```python
from build123d import *

# Parameters (mm, degrees)
SKETCH1_W           = 71.7
SKETCH1_H           = 101.4
BOSS_EXTRUDE1_DEPTH = 11.1
SKETCH5_W           = 87
SKETCH5_H           = 14.461590439
CUT_EXTRUDE1_DEPTH  = 64.5
FILLET2_R           = 1
SKETCH7_R           = 1.5
CUT_EXTRUDE3_DEPTH  = 4
SKETCH10_W          = 8.724930765
SKETCH10_H          = 5.55
CUT_EXTRUDE5_DEPTH  = 10
SKETCH11_W          = 7.2
SKETCH11_H          = 5.55
BOSS_EXTRUDE2_DEPTH = 10
FILLET3_R           = 0.5


with BuildPart() as part:
    # Sketch1 → Boss-Extrude1 (new body)
    with BuildSketch(Plane(origin=(0, 0, 0), x_dir=(1, 0, 0), z_dir=(0, 1, 0))):
        Rectangle(SKETCH1_W, SKETCH1_H)
    extrude(amount=BOSS_EXTRUDE1_DEPTH)

    # Sketch5 → Cut-Extrude1 (cut)
    with BuildSketch(Plane(origin=(35.85, 0, 0), x_dir=(0, 0, -1), z_dir=(1, 0, 0))):
        with Locations((0, 11.23079522)):
            Rectangle(SKETCH5_W, SKETCH5_H)
    extrude(amount=-CUT_EXTRUDE1_DEPTH, mode=Mode.SUBTRACT)

    # Fillet2
    fillet2_edges = [part.edges().sort_by_distance(p)[0] for p in [
        (0, 11.1, -50.7),
        (-35.85, 11.1, 0),
        (-35.85, 0, 0),
        (0, 11.1, 50.7),
        (-35.85, 5.55, -50.7),
        (-35.85, 5.55, 50.7),
    ]]
    fillet(fillet2_edges, radius=FILLET2_R)

    # Sketch7 → Cut-Extrude3 (cut)
    with BuildSketch(Plane(origin=(0, 11.1, 0), x_dir=(1, 0, 0), z_dir=(0, 1, 0))):
        with Locations(Location((-31.75, -6.65790951, 0), (0, 0, 270))):
            Circle(SKETCH7_R)
        with Locations(Location((-31.75, 6.65790951, 0), (0, 0, 90))):
            Circle(SKETCH7_R)
    extrude(amount=-CUT_EXTRUDE3_DEPTH, mode=Mode.SUBTRACT)

    # Sketch10 → Cut-Extrude5 (cut)
    with BuildSketch(Plane(origin=(35.85, 0, 0), x_dir=(0, 0, -1), z_dir=(1, 0, 0))):
        with Locations((-47.862465383, 8.325)):
            Rectangle(SKETCH10_W, SKETCH10_H)
    extrude(amount=-CUT_EXTRUDE5_DEPTH, mode=Mode.SUBTRACT)

    # Sketch11 → Boss-Extrude2 (add)
    with BuildSketch(Plane(origin=(35.85, 0, 0), x_dir=(0, 0, -1), z_dir=(1, 0, 0))):
        with Locations((47.1, 2.775)):
            Rectangle(SKETCH11_W, SKETCH11_H)
    extrude(amount=BOSS_EXTRUDE2_DEPTH)

    # Fillet3
    fillet3_edges = [part.edges().sort_by_distance(p)[0] for p in [
        (-28.65, 4, 0),
        (3.6, 4, -43.5),
        (3.6, 4, 43.5),
        (-28.65, 7.55, -43.5),
        (-28.65, 7.55, 43.5),
        (25.85, 5.55, 47.1),
        (35.85, 5.55, -47.1),
        (35.85, 2, -43.5),
    ]]
    fillet(fillet3_edges, radius=FILLET3_R)


solid = part.part
```
Geometry check sheet. Reference: the model listing, model coordinates, mm. A direction names the side the tool comes from. Give positions to 0.01 mm unless a question says otherwise; leave off trailing zeros. Write each loop counter-clockwise with the first axis right and the second up, starting at its lowest first coordinate (ties: lowest second). Pieces come first, ordered by that corner, then holes.
1) Release check for a two-part mould opening along Z. For faces 1 (the flat face through (-32, 7.1, 7)), 2 (the flat face through (5, 0, 1)), 3 (the flat face through (8, 8, -43.5)), 4 (the flat face through (5, 5, -50.7)) record: pulls with the +Z half, pulls with the -Z half, needs draft (parallel to the pull), parting line crosses it, or undercut.
2) Gauge pin test, flat ends, axial feed: pin 1 (2.5 mm diameter, centred on x = -31.75, z = 6.66, fed in from +Y); pin 2 (3 mm diameter, centred on x = 29.5, z = -9, fed in from +Y); pin 3 (4 mm diameter, centred on y = 8, z = -45.5, fed in from +X). Record the tip position at first contact, or that the pin passes through.
3) Section check A-A, the plane z = 21. Record the boundary of the cut face in (x, y), and give its area (3 significant figures).
4) Material ranges on L1, parallel to Z at x = 27, y = 4.75; L2, parallel to Y at x = -1, z = 30.5; L3, parallel to X at y = 10.25, z = 26, recorded low to high.
5) Section check C-C, the plane x = 40. Record the boundary of the cut face in (y, z).
6) Access from +Z, -Z, +X, -X, +Y, -Y to the whole of each face (thin tool, end or side, straight path). Record for faces 5 (the flat face through (25.85, 9, 47)), 6 (the flat face through (35.85, 9, -47)), 7 (the flat face through (-28.65, 8, 1)), 8 (the flat face through (-32, 7.1, -7)).
7) Section check B-B, the plane x = -31.75. Record the boundary of the cut face in (y, z).
Computed:
1. face 1: undercut
1. face 2: needs draft
1. face 3: undercut
1. face 4: pulls with the -Z half
2. pin 1: stops at y = 7.1
2. pin 2: stops at y = 4
2. pin 3: stops at x = 35.85
3. outline: (-35.85, 1) arc R1 ccw to (-34.85, 0) - (35.85, 0) - (35.85, 4) - (-28.15, 4) arc R0.5 cw to (-28.65, 4.5) - (-28.65, 11.1) - (-34.85, 11.1) arc R1 ccw to (-35.85, 10.1) - close
3. area: 338 mm2
4. L1: z = -50.7 to -43.5, 43.5 to 50.7
4. L2: y = 0 to 4
4. L3: x = -35.84 to -28.65
5. outline: (0, -50.7) - (5.55, -50.7) - (5.55, -43.5) - (0, -43.5) - close
6. face 5: +Z, +X, +Y
6. face 6: +Z, -Z, +X, +Y
6. face 7: +X, +Y
6. face 8: +Y
7. outline: (0, -50.7) - (10.1, -50.7) arc R1 ccw to (11.1, -49.7) - (11.1, -8.16) - (7.1, -8.16) - (7.1, -5.16) - (11.1, -5.16) - (11.1, 5.16) - (7.1, 5.16) - (7.1, 8.16) - (11.1, 8.16) - (11.1, 49.7) arc R1 ccw to (10.1, 50.7) - (0, 50.7) - close
